Verification items for the finished model (mm, model axes). Face numbers are marked on the shaded views. A direction names the side the tool comes from. Give positions to 0.01 mm unless a question says otherwise; leave off trailing zeros. Loops run counter-clockwise (first coordinate to the right, second up) from the corner with the lowest first, then second, coordinate; pieces in that order, holes last. Notation, with made-up numbers: (51, -15) - (98, -15) arc R18 ccw to (98, -2) - close; hole circle Ø8 at (25.25, -38.75). An arc over 180 degrees is marked (long way). One line per question, with ' | ' between items. Start each with the question number.
1. Section check C-C, the plane z = 1. Enter the section's corners in (x, y).
2. Thickness scan on line 1 along X through (y, z) = (4, 4.25); line 2 along Z through (x, y) = (1, 3.5); line 3 along Y through (x, z) = (-2.25, -3.75). Record the ranges inside material, lowest first. Write a range as from..to.
3. Mould release check, pull along Y, two halves, no side actions. Record for the marked faces 1, 2, 3 and 4: +Y half, -Y half, draft (parallel to the pull), parting line (faces both ways), or undercut.
4. Depth check by flat-ended pin: pin 1 Ø1.5 at (y, z) = (-13, -3.5) entering from +X; pin 2 Ø0.5 at (x, y) = (-3.5, -16) entering from +Z; pin 3 Ø0.8 at (x, y) = (-2.5, -9) entering from -Z. Enter the tip coordinate at first touch or a pass-through.
5. Section check B-B, the plane y = -2. Enter the section's corners in (x, z), then the cut area to 3 significant figures.
6. Tool access check on the marked faces 5, 6 and 7. Record the directions out of +Z, -Z, +X, -X, +Y, -Y that give a thin tool (end or side, any length) a straight path to the whole face; none if there is none.
7. Section check A-A, the plane y = -16.75. Enter the section's corners in (x, z) (3 decimals).
from build123d import *

# Parameters (mm, degrees)
BOSS_EXTRUDE1_DEPTH      = 3
BOSS_EXTRUDE2_DEPTH      = 0.7
BOSS_EXTRUDE3_START      = -5.3
BOSS_EXTRUDE3_DEPTH      = 0.7
BOSS_EXTRUDE4_DEPTH      = 1.7
BOSS_EXTRUDE5_DEPTH      = 2.97
BOSS_EXTRUDE6_DEPTH      = 2.5
BOSS_EXTRUDE7_DEPTH      = 0.805
BOSS_EXTRUDE7_DEPTH_BACK = 0.795
SKETCH7_W                = 0.7
SKETCH7_H                = 8.2
CUT_EXTRUDE2_DEPTH       = 0.5
CUT_EXTRUDE3_DEPTH       = 23.844830336
BOSS_EXTRUDE8_DEPTH      = 5.205
INDENT1_START            = -3
INDENT1_DEPTH            = 6
INDENT1_2_DEPTH          = 1.4
INDENT1_START_2          = 1.6
INDENT1_3_OUTLINE_W      = 0.1
INDENT1_3_OUTLINE_H      = 0.4
INDENT1_3_DEPTH          = 1.4
BOSS_EXTRUDE11_START     = 0.05
SKETCH14_W               = 1
SKETCH14_H               = 2
BOSS_EXTRUDE11_DEPTH     = 0.7
BOSS_EXTRUDE11_2_DEPTH   = 0.7
SKETCH15_W               = 1
SKETCH15_H               = 0.7
BOSS_EXTRUDE12_DEPTH     = 0.05
BOSS_EXTRUDE13_REACH     = 25.101
CUT_EXTRUDE4_REACH       = 18.211
SKETCH17_W               = 0.75
SKETCH17_H               = 1.6


# Read off the part's stored shape, not the designer's step: Indent1
with BuildPart() as part:
    # Sketch1 → Boss-Extrude1 (new, symmetric)
    with BuildSketch(Plane(origin=(0, 0, 0), x_dir=(0, 0, -1), z_dir=(1, 0, 0))):
        with BuildLine():
            Line((-4, 5.407024303), (4, 5.407024303))
            ThreePointArc((4, 5.407024303), (5.414213562, 4.821237865), (6, 3.407024303))
            Line((6, 3.407024303), (6, -3.407024303))
            ThreePointArc((6, -3.407024303), (5.881695242, -4.042569102), (5.54262919, -4.592975697))
            ThreePointArc((5.54262919, -4.592975697), (4.399020595, -6.449397799), (4, -8.592975697))
            Line((4, -8.592975697), (4, -18.592975697))
            Line((4, -18.592975697), (4.5, -18.592975697))
            Line((4.5, -18.592975697), (5, -8.592975697))
            ThreePointArc((5, -8.592975697), (5.375406184, -6.605461118), (6.273600288, -4.793172135))
            ThreePointArc((6.273600288, -4.793172135), (6.590990962, -4.132148866), (6.7, -3.407024303))
            Line((6.7, -3.407024303), (6.7, 3.407024303))
            ThreePointArc((6.7, 3.407024303), (5.909188309, 5.316212612), (4, 6.107024303))
            Line((4, 6.107024303), (-4, 6.107024303))
            ThreePointArc((-4, 6.107024303), (-5.909188309, 5.316212612), (-6.7, 3.407024303))
            Line((-6.7, 3.407024303), (-6.7, -3.407024303))
            ThreePointArc((-6.7, -3.407024303), (-6.614300123, -4.08188345), (-6.362640838, -4.7139016))
            ThreePointArc((-6.362640838, -4.7139016), (-5.407997914, -7.026917179), (-5, -9.495706737))
            Line((-5, -9.495706737), (-4.5, -19.495706737))
            Line((-4.5, -19.495706737), (-4, -19.495706737))
            Line((-4, -19.495706737), (-4, -9.495706737))
            ThreePointArc((-4, -9.495706737), (-4.412921237, -6.915479473), (-5.610440713, -4.592975697))
            ThreePointArc((-5.610440713, -4.592975697), (-5.900115974, -4.03117115), (-6, -3.407024303))
            Line((-6, -3.407024303), (-6, 3.407024303))
            ThreePointArc((-6, 3.407024303), (-5.414213562, 4.821237865), (-4, 5.407024303))
        make_face()
    extrude(amount=BOSS_EXTRUDE1_DEPTH, both=True)

    # Sketch2 → Boss-Extrude2 (add)
    with BuildSketch(Plane(origin=(3, 0, 0), x_dir=(0, 0, -1), z_dir=(1, 0, 0))):
        with BuildLine():
            Line((5, -8.592975697), (4.89, -10.792975697))
            Line((4.89, -10.792975697), (-4.935136552, -10.792975697))
            Line((-4.935136552, -10.792975697), (-5, -9.495706737))
            ThreePointArc((-5, -9.495706737), (-5.407997914, -7.026917179), (-6.362640838, -4.7139016))
            ThreePointArc((-6.362640838, -4.7139016), (-6.614300123, -4.08188345), (-6.7, -3.407024303))
            Line((-6.7, -3.407024303), (-6.7, 3.407024303))
            ThreePointArc((-6.7, 3.407024303), (-5.909188309, 5.316212612), (-4, 6.107024303))
            Line((-4, 6.107024303), (4, 6.107024303))
            ThreePointArc((4, 6.107024303), (5.909188309, 5.316212612), (6.7, 3.407024303))
            Line((6.7, 3.407024303), (6.7, -3.407024303))
            ThreePointArc((6.7, -3.407024303), (6.590990962, -4.132148866), (6.273600288, -4.793172135))
            ThreePointArc((6.273600288, -4.793172135), (5.375406184, -6.605461118), (5, -8.592975697))
        make_face()
    extrude(amount=-BOSS_EXTRUDE2_DEPTH)

    # Sketch2<2> → Boss-Extrude3 (add)
    with BuildSketch(Plane(origin=(3, 0, 0), x_dir=(0, 0, -1), z_dir=(1, 0, 0)).offset(BOSS_EXTRUDE3_START)):
        with BuildLine():
            Line((4.89, -10.792975697), (5, -8.592975697))
            ThreePointArc((5, -8.592975697), (5.375406184, -6.605461118), (6.273600288, -4.793172135))
            ThreePointArc((6.273600288, -4.793172135), (6.590990962, -4.132148866), (6.7, -3.407024303))
            Line((6.7, -3.407024303), (6.7, 3.407024303))
            ThreePointArc((6.7, 3.407024303), (5.909188309, 5.316212612), (4, 6.107024303))
            Line((4, 6.107024303), (-4, 6.107024303))
            ThreePointArc((-4, 6.107024303), (-5.909188309, 5.316212612), (-6.7, 3.407024303))
            Line((-6.7, 3.407024303), (-6.7, -3.407024303))
            ThreePointArc((-6.7, -3.407024303), (-6.614300123, -4.08188345), (-6.362640838, -4.7139016))
            ThreePointArc((-6.362640838, -4.7139016), (-5.407997914, -7.026917179), (-5, -9.495706737))
            Line((-5, -9.495706737), (-4.935136552, -10.792975697))
            Line((-4.935136552, -10.792975697), (-4, -10.792975697))
            Line((-4, -10.792975697), (-4, -9.495706737))
            ThreePointArc((-4, -9.495706737), (-4.412921237, -6.915479473), (-5.610440713, -4.592975697))
            ThreePointArc((-5.610440713, -4.592975697), (-5.900115974, -4.03117115), (-6, -3.407024303))
            Line((-6, -3.407024303), (-6, 3.407024303))
            ThreePointArc((-6, 3.407024303), (-5.414213562, 4.821237865), (-4, 5.407024303))
            Line((-4, 5.407024303), (4, 5.407024303))
            ThreePointArc((4, 5.407024303), (5.414213562, 4.821237865), (6, 3.407024303))
            Line((6, 3.407024303), (6, -3.407024303))
            ThreePointArc((6, -3.407024303), (5.881695242, -4.042569102), (5.54262919, -4.592975697))
            ThreePointArc((5.54262919, -4.592975697), (4.399020595, -6.449397799), (4, -8.592975697))
            Line((4, -8.592975697), (4, -10.792975697))
            Line((4, -10.792975697), (4.89, -10.792975697))
        make_face()
        Polygon((4.5, -18.592975697), (4.89, -10.792975697), (4, -10.792975697), (4, -18.592975697), align=None)
        with BuildLine():
            Line((-4, -10.792975697), (4, -10.792975697))
            Line((4, -10.792975697), (4, -8.592975697))
            ThreePointArc((4, -8.592975697), (4.399020595, -6.449397799), (5.54262919, -4.592975697))
            ThreePointArc((5.54262919, -4.592975697), (5.881695242, -4.042569102), (6, -3.407024303))
            Line((6, -3.407024303), (6, 3.407024303))
            ThreePointArc((6, 3.407024303), (5.414213562, 4.821237865), (4, 5.407024303))
            Line((4, 5.407024303), (-4, 5.407024303))
            ThreePointArc((-4, 5.407024303), (-5.414213562, 4.821237865), (-6, 3.407024303))
            Line((-6, 3.407024303), (-6, -3.407024303))
            ThreePointArc((-6, -3.407024303), (-5.900115974, -4.03117115), (-5.610440713, -4.592975697))
            ThreePointArc((-5.610440713, -4.592975697), (-4.412921237, -6.915479473), (-4, -9.495706737))
            Line((-4, -9.495706737), (-4, -10.792975697))
        make_face()
        Polygon((-4, -19.495706737), (-4, -10.792975697), (-4.935136552, -10.792975697), (-4.5, -19.495706737), align=None)
    extrude(amount=-BOSS_EXTRUDE3_DEPTH)

    # Sketch4 → Boss-Extrude4 (add, symmetric)
    with BuildSketch(Plane(origin=(0, 0, 0), x_dir=(0, 0, -1), z_dir=(1, 0, 0))):
        Polygon((3.3, -17.592975697), (4, -17.592975697), (4, -18.592975697), (3.3, -17.792975697), align=None)
    extrude(amount=BOSS_EXTRUDE4_DEPTH, both=True)

    # Sketch5 → Boss-Extrude5 (add)
    with BuildSketch(Plane(origin=(3, 0, 0), x_dir=(0, 0, -1), z_dir=(1, 0, 0))):
        Polygon((-4.495, -19.595706737), (-4.66, -16.295706737), (-4, -16.295706737), (-4, -19.595706737), align=None)
    extrude(amount=BOSS_EXTRUDE5_DEPTH)

    # Sketch6 → Boss-Extrude6 (add)
    with BuildSketch(Plane(origin=(5.97, 0, 0), x_dir=(0, 0, -1), z_dir=(1, 0, 0))):
        Polygon((-4.66, -16.295706737), (-1.51, -16.295706737), (-1.51, -17.795706737), (-3.5, -19.595706737), (-4.495, -19.595706737), align=None)
    extrude(amount=-BOSS_EXTRUDE6_DEPTH)

    # Sketch7 → Boss-Extrude7 (add, two sides: drawn at the far end of the back side and taken through both)
    with BuildSketch(Plane.ZY.offset(3).offset(-BOSS_EXTRUDE7_DEPTH_BACK)):
        with Locations((4.35, -16.492975697)):
            Rectangle(SKETCH7_W, SKETCH7_H)
    extrude(amount=BOSS_EXTRUDE7_DEPTH + BOSS_EXTRUDE7_DEPTH_BACK)

    # Sketch8 → Cut-Extrude2 (cut)
    with BuildSketch(Plane.ZY.offset(3)):
        Polygon((4.7, -15.495706737), (4.7, -12.392975697), (4.855136552, -12.392975697), align=None)
    extrude(amount=-CUT_EXTRUDE2_DEPTH, mode=Mode.SUBTRACT)

    # Sketch9 → Cut-Extrude3 (cut, through all)
    with BuildSketch(Plane.ZY.offset(-3.47)):
        Polygon((2.8, -16.295706737), (1.51, -16.295706737), (1.51, -17.795706737), (3.5, -19.595706737), (2.8, -17.295706737), align=None)
    extrude(amount=-CUT_EXTRUDE3_DEPTH, mode=Mode.SUBTRACT)

    # Sketch10 → Boss-Extrude8 (add)
    with BuildSketch(Plane.ZY.offset(-3)):
        Polygon((4.495, -19.595706737), (4.5, -19.495706737), (4, -19.495706737), (4, -19.595706737), align=None)
    extrude(amount=BOSS_EXTRUDE8_DEPTH)

    # Indent1 outline → Indent1 (cut)
    with BuildSketch(Plane.YZ.offset(INDENT1_START)):
        Polygon((-8.092975697, -2.55), (-8.092975697, 1.85), (-10.692975697, 1.85), (-10.692975697, 2.95), (-10.792975697, 2.95), (-10.792975697, -3.55), (-9.092975697, -3.55), (-9.092975697, -2.55), align=None)
    extrude(amount=INDENT1_DEPTH, mode=Mode.SUBTRACT)

    # Indent1 2 outline → Indent1 2 (cut)
    with BuildSketch(Plane.YZ.offset(INDENT1_START)):
        Polygon((-17.792975697, -3.3), (-17.968374126, -3.453473625), (-17.592975697, -3.487600755), (-17.592975697, -3.3), align=None)
        Polygon((-8.092975697, 2.35), (-9.092975697, 2.35), (-9.092975697, 2.95), (-10.692975697, 2.95), (-10.692975697, 1.85), (-8.092975697, 1.85), align=None)
    extrude(amount=INDENT1_2_DEPTH, mode=Mode.SUBTRACT)

    # Indent1 3 outline → Indent1 3 (cut)
    with BuildSketch(Plane.YZ.offset(INDENT1_START_2)):
        Polygon((-17.792975697, -3.3), (-17.968374126, -3.453473625), (-17.592975697, -3.487600755), (-17.592975697, -3.3), align=None)
        with Locations((-10.742975697, 3.15)):
            Rectangle(INDENT1_3_OUTLINE_W, INDENT1_3_OUTLINE_H)
    extrude(amount=INDENT1_3_DEPTH, mode=Mode.SUBTRACT)



with BuildPart() as body_2:
    # Sketch14 → Boss-Extrude11 (new body)
    with BuildSketch(Plane.ZY.offset(3).offset(BOSS_EXTRUDE11_START)):
        with Locations((1.2, -8.392975697)):
            Rectangle(SKETCH14_W, SKETCH14_H)
    extrude(amount=BOSS_EXTRUDE11_DEPTH)


with BuildPart() as body_3:
    # Sketch14 → Boss-Extrude11 2 (new body)
    with BuildSketch(Plane.ZY.offset(3).offset(BOSS_EXTRUDE11_START)):
        with Locations((-1.4, -8.392975697)):
            Rectangle(SKETCH14_W, SKETCH14_H)
    extrude(amount=BOSS_EXTRUDE11_2_DEPTH)


with BuildPart() as part_1:
    add(part.part)

    add(body_2.part)  # Boss-Extrude12 merges body 2

    add(body_3.part)  # Boss-Extrude12 merges body 3
    # Sketch15 → Boss-Extrude12 (add)
    with BuildSketch(Plane.ZY.offset(3)):
        with Locations((1.2, -7.742975697)):
            Rectangle(SKETCH15_W, SKETCH15_H)
        with Locations((-1.4, -7.742975697)):
            Rectangle(SKETCH15_W, SKETCH15_H)
    extrude(amount=BOSS_EXTRUDE12_DEPTH)

    # Boss-Extrude13: up to this face of the body (flat: up to its plane)
    boss_extrude13_end = Plane(part_1.part.faces().sort_by_distance((-3.390853659, -8.377122039, 1.7))[0])
    # Sketch16 → Boss-Extrude13 (add, up to the picked face)
    with BuildSketch(Plane(origin=(0, 0, -1.9), x_dir=(-1, 0, 0), z_dir=(0, 0, -1)), mode=Mode.PRIVATE) as boss_extrude13_sk1:
        Polygon((3, -7.392975697), (3, -6.642975697), (3.75, -7.392975697), align=None)
    boss_extrude13_tool1 = split(extrude(boss_extrude13_sk1.sketch, amount=-BOSS_EXTRUDE13_REACH, mode=Mode.PRIVATE), bisect_by=boss_extrude13_end, keep=Keep.BOTH, mode=Mode.PRIVATE)
    add(boss_extrude13_tool1.solids().sort_by(Axis((-3.25, -7.142976, -1.9), (0, 0, 1)))[0])

    # Cut-Extrude4: up to this face of the body (flat: up to its plane)
    cut_extrude4_end = Plane(part_1.part.faces().sort_by_distance((-3.375, -7.017975697, -0.1))[0])
    # Sketch17 → Cut-Extrude4 (cut, up to the picked face)
    with BuildSketch(Plane.XZ.offset(7.392975697), mode=Mode.PRIVATE) as cut_extrude4_sk1:
        with Locations((-3.375, -0.1)):
            Rectangle(SKETCH17_W, SKETCH17_H)
    cut_extrude4_tool1 = split(extrude(cut_extrude4_sk1.sketch, amount=-CUT_EXTRUDE4_REACH, mode=Mode.PRIVATE), bisect_by=cut_extrude4_end, keep=Keep.BOTH, mode=Mode.PRIVATE)
    add(cut_extrude4_tool1.solids().sort_by(Axis((-3.375, -7.392976, -0.1), (0, 1, 0)))[0], mode=Mode.SUBTRACT)


solid = part_1.part
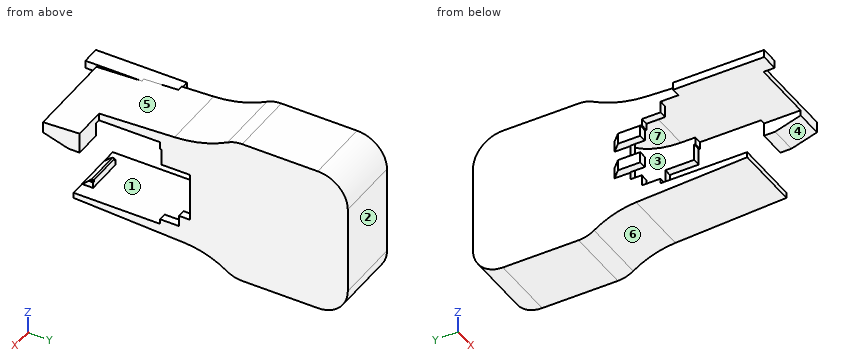
Results list:
1) outline: (-3.75, -9.39) - (-3.05, -9.39) - (-3.05, -8.09) - (-2.3, -8.09) - (-2.3, 5.41) - (2.3, 5.41) - (2.3, -8.09) - (3, -8.09) - (3, 6.11) - (-3, 6.11) - (-3, -6.64) - (-3.75, -7.39) - close
2) line 1: -3..-2.3, 2.3..3 | line 2: -6.7..-6, 6..6.7 | line 3: 5.41..6.11
3) face 1: undercut | face 2: +Y half | face 3: undercut | face 4: -Y half
4) pin 1: x = 3 | pin 2: z = 4.7 | pin 3: z = -5
5) outline: (-3, -6.7) - (3, -6.7) - (3, 6.7) - (-3, 6.7) - close; hole (-2.3, -6) - (2.3, -6) - (2.3, 6) - (-2.3, 6) - close | area: 25.2 mm²
6) face 5: +Z, +X, -Y | face 6: -Z, +X, -X, -Y | face 7: none
7) outline: (-3.805, 4) - (3.47, 4) - (3.47, 2.8) - (5.97, 2.8) - (5.97, 4.637) - (-2.205, 4.637) - (-2.205, 4.7) - (-3.805, 4.7) - close; (-3, -4.592) - (3, -4.592) - (3, -4) - (-3, -4) - close
